Read the model definition and answer for the solid it produces. Units are mm, in the model's axes. A direction names the side the tool comes from. Give positions to 0.01 mm unless a question says otherwise; leave off trailing zeros. Order: outer loops, then holes, each group sorted by start corner. A loop starts at its lowest first (then second) coordinate and runs counter-clockwise, first axis right, second up. Notation, with made-up numbers: (-28.5, 27) -> (0.5, 27) arc R16 cw to (0.5, 40) -> close; hole circle Ø9 at (45.25, 30). An arc over 180 degrees is marked (long way). Answer as CSV lines item,"result". Start each with the question number.
1) Flat-ended cylindrical pins translate along their axes: pin 1 Ø1 at (x, z) = (7, -2) entering from +Y; pin 2 Ø3 at (x, y) = (3, 14.5) entering from -Z; pin 3 Ø1 at (y, z) = (16, -1.5) entering from -X; pin 4 Ø9 at (x, y) = (13.25, 22.95) entering from +Z. Find the tip coordinate at first contact, or state that the pin passes through.
2) The mould has two halves that part along X. Classify faces 1 (the face through (-7.912, -35.632, -1.479)), 2 (the face through (18.02, 24.45, -0.99)), 3 (the face through (16, -8, -3)): +X half, -X half, draft (parallel to the pull), parting line (faces both ways), or undercut.
3) Find section A-A (y = 0). Determine the outline of the cut face in (x, z) (3 decimals), and give its area (3 significant figures).
4) Straight lines are drawn through the part: L1, parallel to Y at x = 13.25, z = -2.3; L2, parallel to X at y = -20.5, z = -0.15; L3, parallel to Y at x = -11, z = -1.3. For each, find the intervals that lie inside material, in ascending order. Write a range as from..to.
5) For faces 4 (the face through (-11.41, -21.26, -2.51)), 5 (the face through (-8.48, 24.45, -0.99)), determine the directions among +Z, -Z, +X, -X, +Y, -Y from which every point of the face is accessible in a straight line to the end or side of a thin tool.
6) Find section C-C (z = -2.45). Determine the outline of the cut face in (x, y) (3 decimals), and give its area (3 significant figures).
7) Find section D-D (x = -26.5). Determine the outline of the cut face in (y, z) (3 decimals), and give its area (3 significant figures).
8) Find section B-B (x = 0). Determine the outline of the cut face in (y, z).
```python
from build123d import *

# Parameters (mm, degrees)
F0_R           = 36.5
F0_R_2         = 16.5
F1_DEPTH       = 3
F2_D           = 5
F2_CBORE_D     = 10
F2_CBORE_DEPTH = 2
F3_D           = 5.85
F3_CBORE_D     = 10
F3_CBORE_DEPTH = 1.3


with BuildPart() as f1:
    # F0 (on Top) → F1 (new body)
    with BuildSketch(Plane.XY):
        Circle(F0_R)
        Circle(F0_R_2, mode=Mode.SUBTRACT)
    extrude(amount=-F1_DEPTH)

    # F2 (through all)
    with Locations(Plane.XY):
        with Locations((-13.25, 22.949673), (13.25, 22.949673), (-13.25, -22.949673), (13.25, -22.949673)):
            CounterBoreHole(F2_D / 2, F2_CBORE_D / 2, F2_CBORE_DEPTH)

    # F3 (through all)
    with Locations(Plane.XY):
        with Locations((-26.5, 0), (26.5, 0)):
            CounterBoreHole(F3_D / 2, F3_CBORE_D / 2, F3_CBORE_DEPTH)


solid = f1.part
```
Findings below:
1,pin 1,"y = 35.92"
1,pin 2,"through"
1,pin 3,"x = -33.05"
1,pin 4,"z = -2"
2,face 1,"parting line"
2,face 2,"undercut"
2,face 3,"draft"
3,outline,"(-36.5, -3) -> (-29.425, -3) -> (-29.425, -1.3) -> (-31.5, -1.3) -> (-31.5, 0) -> (-36.5, 0) -> close; (-23.575, -3) -> (-16.5, -3) -> (-16.5, 0) -> (-21.5, 0) -> (-21.5, -1.3) -> (-23.575, -1.3) -> close; (16.5, -3) -> (23.575, -3) -> (23.575, -1.3) -> (21.5, -1.3) -> (21.5, 0) -> (16.5, 0) -> close; (29.425, -3) -> (36.5, -3) -> (36.5, 0) -> (31.5, 0) -> (31.5, -1.3) -> (29.425, -1.3) -> close"
3,area,"74.1 mm²"
4,L1,"-34.01..-25.45, -20.45..-9.83, 9.83..20.45, 25.45..34.01"
4,L2,"-30.2..-17.61, -8.89..8.89, 17.61..30.2"
4,L3,"-34.8..-27.41, -18.48..-12.3, 12.3..18.48, 27.41..34.8"
5,face 4,"+Z, -Z"
5,face 5,"+Z"
6,outline,"circle Ø73 at (0, 0); hole circle Ø5.85 at (-26.5, 0); hole circle Ø33 at (0, 0); hole circle Ø5 at (-13.25, -22.95); hole circle Ø5 at (-13.25, 22.95); hole circle Ø5 at (13.25, -22.95); hole circle Ø5 at (13.25, 22.95); hole circle Ø5.85 at (26.5, 0)"
6,area,"3,200 mm²"
7,outline,"(-25.1, -3) -> (-2.925, -3) -> (-2.925, -1.3) -> (-5, -1.3) -> (-5, 0) -> (-25.1, 0) -> close; (2.925, -3) -> (25.1, -3) -> (25.1, 0) -> (5, 0) -> (5, -1.3) -> (2.925, -1.3) -> close"
7,area,"128 mm²"
8,outline,"(-36.5, -3) -> (-16.5, -3) -> (-16.5, 0) -> (-36.5, 0) -> close; (16.5, -3) -> (36.5, -3) -> (36.5, 0) -> (16.5, 0) -> close"
